For this review, take the finished solid that the model builds, in its own axes (mm). Round coordinates to 2 decimals unless told otherwise and drop trailing zeros. Order: outer loops, then holes, each group sorted by start corner. A loop starts at its lowest first (then second) coordinate and runs counter-clockwise, first axis right, second up.
```python
from build123d import *

# Parameters (mm, degrees)
SKETCH1_W           = 35
SKETCH1_H           = 35
BOSS_EXTRUDE1_DEPTH = 4
SKETCH3_R           = 1.6
DOWEL_CUT_DEPTH     = 26.069902273
SKETCH2_R           = 2.5
SCREW_CUT_DEPTH     = 26.069902273


with BuildPart() as part:
    # Sketch1 → Boss-Extrude1 (new body)
    with BuildSketch(Plane.XY):
        Rectangle(SKETCH1_W, SKETCH1_H)
    extrude(amount=BOSS_EXTRUDE1_DEPTH)

    # Sketch3 → Dowel cut (cut, through all)
    with BuildSketch(Plane.XY.offset(4)):
        with Locations((-12.5, 12.5)):
            Circle(SKETCH3_R)
        with Locations((12.5, 12.5)):
            Circle(SKETCH3_R)
        with Locations((12.5, -12.5)):
            Circle(SKETCH3_R)
        with Locations((-12.5, -12.5)):
            Circle(SKETCH3_R)
    extrude(amount=-DOWEL_CUT_DEPTH, mode=Mode.SUBTRACT)

    # Sketch2 → Screw cut (cut, through all)
    with BuildSketch(Plane.XY.offset(4)):
        Circle(SKETCH2_R)
    extrude(amount=-SCREW_CUT_DEPTH, mode=Mode.SUBTRACT)


solid = part.part
```
Q1. Clearance check with a flat-ended pin moving along its axis: pin 1 (3 mm diameter, centred on x = -12.5, y = -12.5, fed in from -Z). State where the tip first meets the part, or that it passes through.
Q2. Take a section at A-A, the plane x = 0. State the section outline as (y, z) points.
Q3. Take a section at B-B, the plane x = 12.5. State the section outline as (y, z) points.
Q4. Take a section at D-D, the plane z = 2.75. State the section outline as (x, y) points, plus the area to 3 significant figures.
Q5. Wall thickness on line 1 (Y direction, x = -12.5, z = 2.85); line 2 (Y direction, x = -11.5, z = 2.45); line 3 (X direction, y = -13, z = 2.7): over which ranges is each line inside the solid? List them lowest first.
Working result:
1. pin 1: passes through
2. outline: (-17.5, 0) - (-2.5, 0) - (-2.5, 4) - (-17.5, 4) - close; (2.5, 0) - (17.5, 0) - (17.5, 4) - (2.5, 4) - close
3. outline: (-17.5, 0) - (-14.1, 0) - (-14.1, 4) - (-17.5, 4) - close; (-10.9, 0) - (10.9, 0) - (10.9, 4) - (-10.9, 4) - close; (14.1, 0) - (17.5, 0) - (17.5, 4) - (14.1, 4) - close
4. outline: (-17.5, -17.5) - (17.5, -17.5) - (17.5, 17.5) - (-17.5, 17.5) - close; hole circle Ø3.2 at (-12.5, -12.5); hole circle Ø3.2 at (-12.5, 12.5); hole circle Ø5 at (0, 0); hole circle Ø3.2 at (12.5, -12.5); hole circle Ø3.2 at (12.5, 12.5)
4. area: 1,170 mm2
5. line 1: y = -17.5 to -14.1, -10.9 to 10.9, 14.1 to 17.5
5. line 2: y = -17.5 to -13.75, -11.25 to 11.25, 13.75 to 17.5
5. line 3: x = -17.5 to -14.02, -10.98 to 10.98, 14.02 to 17.5
